Could you check a few things on this model? Use its own coordinates, in mm. Face numbers are marked on the shaded views. Round coordinates to 2 decimals unless told otherwise and drop trailing zeros. Write each loop counter-clockwise with the first axis right and the second up, starting at its lowest first coordinate (ties: lowest second). Pieces come first, ordered by that corner, then holes. Notation, with made-up numbers: (49.25, 37) -> (76.25, 37) arc R28 cw to (76.25, 61) -> close; hole circle Ø8 at (78, -11.5). An arc over 180 degrees is marked (long way). Answer in a Markdown table with one row per item.
from build123d import *

# Parameters (mm, degrees)
BOSS_EXTRUDE1_DEPTH = 8.89
FILLET1_R           = 4.191
FILLET2_R           = 1.27


with BuildPart() as part:
    # Sketch1 → Boss-Extrude1 (new body)
    with BuildSketch(Plane(origin=(0, 0, 0), x_dir=(1, 0, 0), z_dir=(0, 1, 0))):
        with BuildLine():
            Line((-8.89, 3.81), (-8.89, 62.23))
            ThreePointArc((-8.89, 62.23), (-5.170256121, 71.210256121), (3.81, 74.93))
            Line((3.81, 74.93), (62.23, 74.93))
            ThreePointArc((62.23, 74.93), (71.210256121, 71.210256121), (74.93, 62.23))
            Line((74.93, 62.23), (74.93, 3.81))
            ThreePointArc((74.93, 3.81), (71.210256121, -5.170256121), (62.23, -8.89))
            Line((62.23, -8.89), (3.81, -8.89))
            ThreePointArc((3.81, -8.89), (-5.170256121, -5.170256121), (-8.89, 3.81))
        make_face()
        with BuildLine():
            Line((3.81, 0), (62.23, 0))
            ThreePointArc((62.23, 0), (64.924076836, 1.115923164), (66.04, 3.81))
            Line((66.04, 3.81), (66.04, 62.23))
            ThreePointArc((66.04, 62.23), (64.924076836, 64.924076836), (62.23, 66.04))
            Line((62.23, 66.04), (3.81, 66.04))
            ThreePointArc((3.81, 66.04), (1.115923164, 64.924076836), (0, 62.23))
            Line((0, 62.23), (0, 3.81))
            ThreePointArc((0, 3.81), (1.115923164, 1.115923164), (3.81, 0))
        make_face(mode=Mode.SUBTRACT)
    extrude(amount=BOSS_EXTRUDE1_DEPTH)

    # Fillet1
    fillet1_edges = [part.edges().sort_by_distance(p)[0] for p in [
        (71.210256121, 8.89, 5.170256121),
        (74.93, 8.89, -33.02),
        (71.210256121, 8.89, -71.210256121),
        (33.02, 8.89, -74.93),
        (-5.170256121, 8.89, -71.210256121),
        (-8.89, 8.89, -33.02),
        (1.115923164, 8.89, -1.115923164),
        (33.02, 8.89, 0),
        (64.924076836, 8.89, -1.115923164),
        (66.04, 8.89, -33.02),
        (64.924076836, 8.89, -64.924076836),
        (33.02, 8.89, -66.04),
        (1.115923164, 8.89, -64.924076836),
        (0, 8.89, -33.02),
        (-5.170256121, 8.89, 5.170256121),
        (33.02, 8.89, 8.89),
    ]]
    fillet(fillet1_edges, radius=FILLET1_R)

    # Fillet2
    fillet2_edges = [part.edges().sort_by_distance(p)[0] for p in [
        (33.02, 0, 8.89),
        (-5.170256121, 0, 5.170256121),
        (1.115923164, 0, -1.115923164),
        (33.02, 0, 0),
        (64.924076836, 0, -1.115923164),
        (66.04, 0, -33.02),
        (64.924076836, 0, -64.924076836),
        (33.02, 0, -66.04),
        (1.115923164, 0, -64.924076836),
        (0, 0, -33.02),
        (-8.89, 0, -33.02),
        (-5.170256121, 0, -71.210256121),
        (33.02, 0, -74.93),
        (71.210256121, 0, -71.210256121),
        (74.93, 0, -33.02),
        (71.210256121, 0, 5.170256121),
    ]]
    fillet(fillet2_edges, radius=FILLET2_R)


solid = part.part
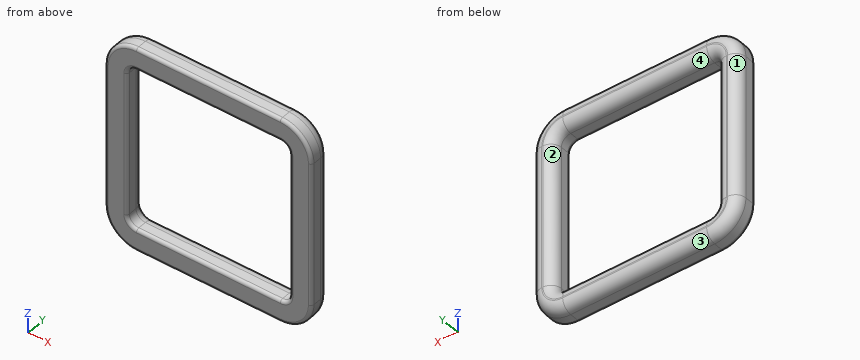
1) For pin 1 (5 mm diameter, centred on x = 3.5, y = 8, fed in from -Z), with a flat end and sliding along its axis, tell me the tip position at first contact or that it passes through.
Findings:
| item | result |
|---|---|
| pin 1 | stops at z = -74.85 |
2) Imagine slicing it at A-A, the plane x = 56. Please give me the cut outline in (y, z), plus the area to 3 significant figures.
Findings:
| item | result |
|---|---|
| outline | (0, -73.66) arc R1.27 ccw to (1.27, -74.93) -> (4.7, -74.93) arc R4.19 ccw to (8.89, -70.74) -> (8.89, -70.23) arc R4.19 ccw to (4.7, -66.04) -> (1.27, -66.04) arc R1.27 ccw to (0, -67.31) -> close; (0, 1.27) arc R1.27 ccw to (1.27, 0) -> (4.7, 0) arc R4.19 ccw to (8.89, 4.19) -> (8.89, 4.7) arc R4.19 ccw to (4.7, 8.89) -> (1.27, 8.89) arc R1.27 ccw to (0, 7.62) -> close |
| area | 142 mm^2 |
3) Thinking about a two-plate mould opening in Z: for the marked faces 1, 2, 3 and 4, which applies, +Z half, -Z half, draft (parallel to the pull), parting line (faces both ways), or undercut?
Findings:
| item | result |
|---|---|
| face 1 | draft |
| face 2 | undercut |
| face 3 | -Z half |
| face 4 | undercut |
4) Imagine slicing it at B-B, the plane z = -52.5. Please give me the cut outline in (x, y).
Findings:
| item | result |
|---|---|
| outline | (-8.89, 1.27) arc R1.27 ccw to (-7.62, 0) -> (-1.27, 0) arc R1.27 ccw to (0, 1.27) -> (0, 4.7) arc R4.19 ccw to (-4.19, 8.89) -> (-4.7, 8.89) arc R4.19 ccw to (-8.89, 4.7) -> close; (66.04, 1.27) arc R1.27 ccw to (67.31, 0) -> (73.66, 0) arc R1.27 ccw to (74.93, 1.27) -> (74.93, 4.7) arc R4.19 ccw to (70.74, 8.89) -> (70.23, 8.89) arc R4.19 ccw to (66.04, 4.7) -> close |
5) Please list where these lines run through material, in increasing order: line 1 (Z direction, x = 20, y = 2.75); line 2 (X direction, y = 4.5, z = -33); line 3 (X direction, y = 5, z = -61).
Findings:
| item | result |
|---|---|
| line 1 | z = -74.93 to -66.04, 0 to 8.89 |
| line 2 | x = -8.89 to 0, 66.04 to 74.93 |
| line 3 | x = -8.88 to -0.01, 66.05 to 74.92 |
6) Imagine slicing it at C-C, the plane y = 7.75. Please give me the cut outline in (x, z).
Findings:
| item | result |
|---|---|
| outline | (-7.57, -62.23) arc R11.38 ccw to (3.81, -73.61) -> (62.23, -73.61) arc R11.38 ccw to (73.61, -62.23) -> (73.61, -3.81) arc R11.38 ccw to (62.23, 7.57) -> (3.81, 7.57) arc R11.38 ccw to (-7.57, -3.81) -> close; hole (-1.32, -62.23) arc R5.13 ccw to (3.81, -67.36) -> (62.23, -67.36) arc R5.13 ccw to (67.36, -62.23) -> (67.36, -3.81) arc R5.13 ccw to (62.23, 1.32) -> (3.81, 1.32) arc R5.13 ccw to (-1.32, -3.81) -> close |
